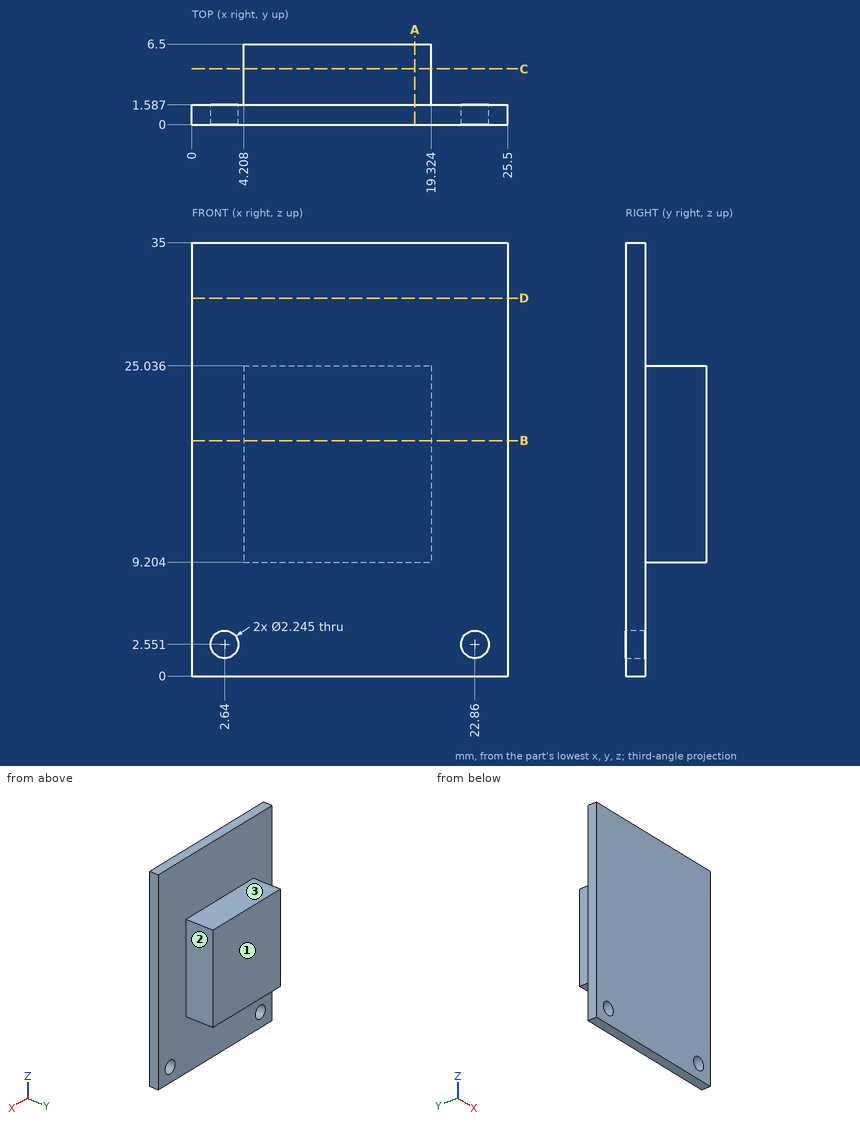
Here's the drawing with two shaded views (mm, measured from the low corner). I have some questions. A direction names the side the tool comes from. Give positions to 0.01 mm unless a question says otherwise; leave off trailing zeros. Loops run counter-clockwise (first coordinate to the right, second up) from the corner with the lowest first, then second, coordinate; pieces in that order, holes last. Notation, with made-up numbers: M 85,6.25 L 131,6.25 A14 cw 131,23.25 Z; hole C 31,-31 d6. An arc over 180 degrees is marked long. One line per item, written item: value.
(1) Suppose I cut it at C-C on y = 4.5. List the corners of the cut face in (x, z) for me (1 decimal).
Returned:
outline: M 4.2,9.2 L 19.3,9.2 L 19.3,25 L 4.2,25 Z
(2) Suppose I cut it at B-B on z = 19. List the corners of the cut face in (x, y) for me (1 decimal).
Returned:
outline: M 0,0 L 25.5,0 L 25.5,1.6 L 19.3,1.6 L 19.3,6.5 L 4.2,6.5 L 4.2,1.6 L 0,1.6 Z
(3) Which directions (+Z, -Z, +X, -X, +Y, -Y) give clear straight access to the entire face, cutting with the end or side of a thin tool? Please do the marked faces 1, 2 and 3.
Returned:
face 1: +Z, -Z, +X, -X, +Y
face 2: +Z, -Z, +X, +Y
face 3: +Z, +X, -X, +Y
(4) Suppose I cut it at D-D on z = 30.5. List the corners of the cut face in (x, y) for me.
Returned:
outline: M 0,0 L 25.5,0 L 25.5,1.59 L 0,1.59 Z
(5) Suppose I cut it at A-A on x = 18. List the corners of the cut face in (y, z) for me (1 decimal).
Returned:
outline: M 0,0 L 1.6,0 L 1.6,9.2 L 6.5,9.2 L 6.5,25 L 1.6,25 L 1.6,35 L 0,35 Z
(6) Will these pins go through, and if not, where does the flat tip stop? pin 1 (1.3 mm diameter, centred on x = 22.86, z = 2.55, fed in from -Y); pin 2 (1 mm diameter, centred on x = 8.5, y = 2.5, fed in from +Z); pin 3 (1 mm diameter, centred on y = 4, z = 23, fed in from -X); pin 4 (3.5 mm diameter, centred on x = 2.64, z = 2.55, fed in from +Y).
Returned:
pin 1: through
pin 2: z = 25.04
pin 3: x = 4.21
pin 4: y = 1.59
(7) I need wall thicknesses on line 1 (X direction, y = 1.25, z = 2); line 2 (Y direction, x = 15, z = 31.5); line 3 (X direction, y = 2, z = 10.5) (1 decimal). Which ranges of each line are inside material? Lowest first, please.
Returned:
line 1: 0 to 1.66, 3.62 to 21.88, 23.84 to 25.5
line 2: 0 to 1.59
line 3: 4.2 to 19.3
